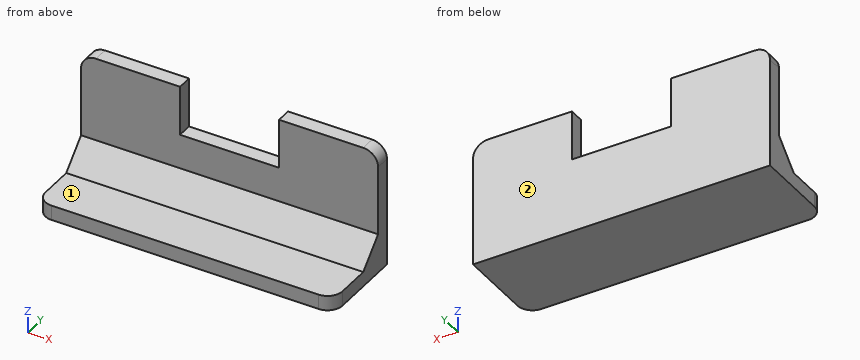
```python
from build123d import *

# Parameters (mm, degrees)
SKETCH1_W           = 60
SKETCH1_H           = 3
BOSS_EXTRUDE1_DEPTH = 25
SKETCH2_W           = 60
SKETCH2_H           = 3
BOSS_EXTRUDE2_DEPTH = 15
SKETCH3_W           = 20
SKETCH3_H           = 10
CUT_EXTRUDE1_DEPTH  = 42.833001327
FILLET1_R           = 3
CHAMFER1_SIZE       = 5


with BuildPart() as part:
    # Sketch1 → Boss-Extrude1 (new body)
    with BuildSketch(Plane.XY):
        with Locations((0, 158.5)):
            Rectangle(SKETCH1_W, SKETCH1_H)
    extrude(amount=BOSS_EXTRUDE1_DEPTH)

    # Sketch2 → Boss-Extrude2 (add)
    with BuildSketch(Plane.XZ.offset(-157)):
        with Locations((0, 1.5)):
            Rectangle(SKETCH2_W, SKETCH2_H)
    extrude(amount=BOSS_EXTRUDE2_DEPTH)

    # Sketch3 → Cut-Extrude1 (cut, through all)
    with BuildSketch(Plane.XZ.offset(-157)):
        with Locations((0, 20)):
            Rectangle(SKETCH3_W, SKETCH3_H)
    extrude(amount=-CUT_EXTRUDE1_DEPTH, mode=Mode.SUBTRACT)

    # Fillet1
    fillet1_edges = [part.edges().sort_by_distance(p)[0] for p in [
        (30, 158.5, 25),
        (-30, 142, 1.5),
        (30, 142, 1.5),
        (-30, 158.5, 25),
    ]]
    fillet(fillet1_edges, radius=FILLET1_R)

    # Chamfer1
    chamfer1_edges = [part.edges().sort_by_distance(p)[0] for p in [
        (0, 157, 3),
    ]]
    chamfer(chamfer1_edges, length=CHAMFER1_SIZE)


solid = part.part
```
Here's how the part is built. I have some questions about the finished solid (model axes, mm). Face numbers are marked on the shaded views. A direction names the side the tool comes from. Coordinates: 2 decimals unless noted, no trailing zeros. Order: outer loops, then holes, each group sorted by start corner. A loop starts at its lowest first (then second) coordinate and runs counter-clockwise, first axis right, second up.
Item 1: I need wall thicknesses on probe 1 along X at (y, z) = (158, 16); probe 2 along Z at (x, y) = (3.5, 150.25); probe 3 along Y at (x, z) = (19, 14). Which ranges of each line are inside material? Lowest first, please.
Response values:
probe 1: x = -30 to -10, 10 to 30
probe 2: z = 0 to 3
probe 3: y = 157 to 160
Item 2: If we section it at A-A, the plane x = 12.5: List the corners of the cut face in (y, z) for me, then the cut area to 4 significant figures.
Response values:
outline: (142, 0) - (160, 0) - (160, 25) - (157, 25) - (157, 8) - (152, 3) - (142, 3) - close
area: 132.5 mm2
Item 3: I'm going to push flat-ended pins straight in: pin 1 Ø8 at (x, y) = (-13, 144.5) entering from +Z; pin 2 Ø2.5 at (x, y) = (0.5, 158) entering from +Z; pin 3 Ø6 at (x, z) = (-13, 18) entering from -Y. Where does each tip first touch, or does it pass through?
Response values:
pin 1: stops at z = 3
pin 2: stops at z = 15
pin 3: stops at y = 157
Item 4: Which directions (+Z, -Z, +X, -X, +Y, -Y) give clear straight access to the entire face, cutting with the end or side of a thin tool? Please do the marked faces 1 and 2.
Response values:
face 1: +Z, +X, -X, -Y
face 2: +Z, -Z, +X, -X, +Y
Item 5: If we section it at B-B, the plane y = 158.25: List the corners of the cut face in (x, z) for me.
Response values:
outline: (-30, 0) - (30, 0) - (30, 22) arc R3 ccw to (27, 25) - (10, 25) - (10, 15) - (-10, 15) - (-10, 25) - (-27, 25) arc R3 ccw to (-30, 22) - close
Item 6: If we section it at D-D, the plane z = 11.25: List the corners of the cut face in (x, y) for me.
Response values:
outline: (-30, 157) - (30, 157) - (30, 160) - (-30, 160) - close
Item 7: If we section it at C-C, the plane z = 23.5: List the corners of the cut face in (x, y) for me, then the cut area to 3 significant figures.
Response values:
outline: (-29.6, 157) - (-10, 157) - (-10, 160) - (-29.6, 160) - close; (10, 157) - (29.6, 157) - (29.6, 160) - (10, 160) - close
area: 118 mm2
